Geometry check sheet. Reference: the model listing, model coordinates, mm. Face numbers are marked on the shaded views. A direction names the side the tool comes from. Coordinates: 2 decimals unless noted, no trailing zeros. Order: outer loops, then holes, each group sorted by start corner. A loop starts at its lowest first (then second) coordinate and runs counter-clockwise, first axis right, second up. Notation, with made-up numbers: (33.5, 70) - (86.5, 70) arc R29 cw to (86.5, 94) - close; hole circle Ø3 at (81, 68). An arc over 180 degrees is marked (long way). One line per item, written item: value. Start each with the question number.
```python
from build123d import *

# Parameters (mm, degrees)
SKETCH_W           = 18.5
SKETCH_H           = 18.5
SKETCH_R           = 8.15
PAD_DEPTH          = 4
SKETCH001_W        = 18.5
SKETCH001_H        = 18.5
PAD001_DEPTH       = 3
SKETCH002_R        = 9.25
SKETCH003_R        = 5.4
SKETCH005_R        = 5.4
PAD002_DEPTH       = 2
CHAMFER_SIZE       = 1.5
CHAMFER001_SIZE    = 1.5
POCKET_DEPTH       = 102.726887
POLARPATTERN_COUNT = 4
SKETCH007_R        = 4.4
SKETCH008_R        = 5.4
SKETCH009_W        = 9
SKETCH009_H        = 1
PAD003_DEPTH       = 1
SKETCH012_R        = 0.5655
SKETCH012_W        = 3.231
SKETCH012_H        = 0.497
POCKET001_DEPTH    = 18.501
POCKET002_DEPTH    = 13.751


with BuildPart() as part:
    # Sketch → Pad (new body)
    with BuildSketch(Plane.XY):
        Rectangle(SKETCH_W, SKETCH_H)
        Circle(SKETCH_R, mode=Mode.SUBTRACT)
    extrude(amount=PAD_DEPTH)

    # Sketch001 (on Face7 of Pad) → Pad001 (join)
    with BuildSketch(Plane.XY.offset(4)):
        Rectangle(SKETCH001_W, SKETCH001_H)
    extrude(amount=PAD001_DEPTH)

    # Sketch002 (on Face10 of Pad001) → AdditiveLoft section 0
    with BuildSketch(Plane.XY.offset(7)):
        Circle(SKETCH002_R)
    # Sketch003 (on Face10 of Pad001) → AdditiveLoft section 1
    with BuildSketch(Plane.XY.offset(31)):
        Circle(SKETCH003_R)
    loft()

    # Sketch005 (on Face17 of AdditiveLoft) → Pad002 (join)
    with BuildSketch(Plane.XY.offset(31)):
        Circle(SKETCH005_R)
    extrude(amount=PAD002_DEPTH)

    # Chamfer
    chamfer_edges = [part.edges().sort_by_distance(p)[0] for p in [
        (-9.25, -9.25, 5.5),
        (-9.25, -9.25, 2),
        (9.25, -9.25, 5.5),
        (9.25, -9.25, 2),
        (9.25, 9.25, 2),
        (9.25, 9.25, 5.5),
        (-9.25, 9.25, 5.5),
        (-9.25, 9.25, 2),
    ]]
    chamfer(chamfer_edges, length=CHAMFER_SIZE)

    # Chamfer001
    chamfer001_edges = [part.edges().sort_by_distance(p)[0] for p in [
        (8.5, -8.5, 7),
        (-8.5, -8.5, 7),
        (-8.5, 8.5, 7),
        (8.5, 8.5, 7),
    ]]
    chamfer(chamfer001_edges, length=CHAMFER001_SIZE)

    # Sketch006 (on Face19 of Chamfer001) → Pocket (cut, through all)
    with BuildSketch(Plane.YZ.offset(9.25)):
        Polygon((0, 31), (-2.7, 7), (2.7, 7), align=None)
    pocket = extrude(amount=-POCKET_DEPTH, mode=Mode.SUBTRACT)

    # PolarPattern: Pocket ×4 about axis
    polarpattern_axis = Axis((0, 0, 0), (0, 0, 1))
    for i in range(1, POLARPATTERN_COUNT):
        add(pocket.rotate(polarpattern_axis, i * 360 / POLARPATTERN_COUNT), mode=Mode.SUBTRACT)

    # Sketch007 (on Face47 of PolarPattern) → AdditiveLoft001 section 0
    with BuildSketch(Plane.XY.offset(33)):
        Circle(SKETCH007_R)
    # Sketch008 → AdditiveLoft001 section 1
    with BuildSketch(Plane.XY.offset(35)):
        Circle(SKETCH008_R)
    loft()

    # Sketch009 (on Face56 of AdditiveLoft001) → Pad003 (join)
    with BuildSketch(Plane.XY.offset(35)):
        Rectangle(SKETCH009_W, SKETCH009_H)
    extrude(amount=PAD003_DEPTH)

    # Sketch010 (on Face59 of Pad003) → AdditiveLoft002 section 0
    with BuildSketch(Plane.YZ.offset(4.5)):
        Polygon((-3, 35), (-4.75, 43), (4.75, 43), (3, 35), align=None)
    # Sketch011 → AdditiveLoft002 section 1
    with BuildSketch(Plane(origin=(-6, 0, 0), x_dir=(0, -1, 0), z_dir=(-1, 0, 0))):
        Polygon((-1.5, 37.4), (1.5, 37.4), (1, 35), (-1, 35), align=None)
    loft()

    # Sketch012 (on Face43 of AdditiveLoft002) → Pocket001 (cut, through all)
    with BuildSketch(Plane.XZ.offset(9.25)):
        with Locations((1.06, 38.921)):
            Circle(SKETCH012_R)
        with Locations((-4.9245, 36.0185)):
            Rectangle(SKETCH012_W, SKETCH012_H)
    extrude(amount=-POCKET001_DEPTH, mode=Mode.SUBTRACT)

    # Sketch013 (on Face62 of Pocket001) → Pocket002 (cut, through all)
    with BuildSketch(Plane.YZ.offset(4.5)):
        Polygon((0, 44.847), (5.530097, 43.207534), (0, 41.847), (-5.530097, 43.207534), align=None)
    extrude(amount=-POCKET002_DEPTH, mode=Mode.SUBTRACT)


solid = part.part
```
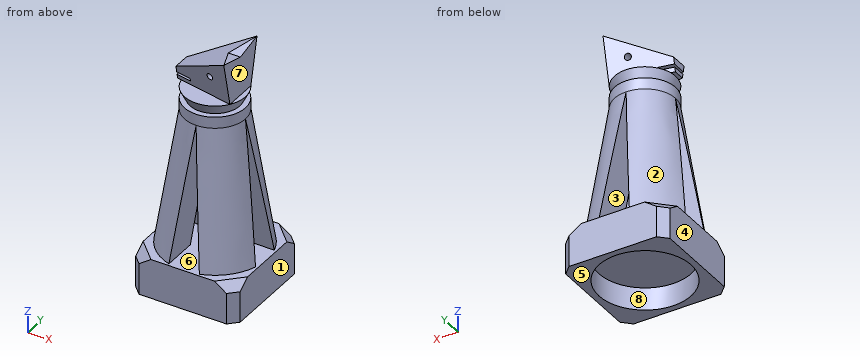
Q1. Material ranges on probe 1 along Y at (x, z) = (0, 3.2); probe 2 along Z at (x, y) = (5.5, 0); probe 3 along X at (y, z) = (5.25, 22.5), recorded low to high.
Q2. Cross-section at B-B, the plane y = 0.5. Count the separate pieces of the cut face and the enclosed holes in it, and give its area (3 significant figures).
Q3. Cross-section at C-C, the plane z = 33.5. Enter the section's corners in (x, y).
Q4. Gauge pin test, flat ends, axial feed: P1, Ø8, axis at x = 1.5, y = 3, coming from the -Z side; P2, Ø1.3, axis at x = -5, y = 0.5, coming from the +Z side; P3, Ø5.5, axis at x = 0, y = 0.5, coming from the +Z side; P4, Ø6, axis at x = 4.5, y = 2, coming from the +Z side. Record the tip position at first contact, or that the pin passes through.
Q5. Cross-section at A-A, the plane z = 18. Enter the section's corners in (x, y), and give its area (3 significant figures).
Q6. Set-up check for the marked faces 4, 5, 6, 7 and 8: record each of +Z, -Z, +X, -X, +Y, -Y from which the full face is reachable in a straight line by a thin tool's end or side.
Q7. Release check for a two-part mould opening along X. For the marked faces 1, 2 and 3 record: released by +X, released by -X, zero draft, split by the parting line, or undercut.
Check result:
1. probe 1: y = -9.25 to -8.15, 8.15 to 9.25
1. probe 2: z = 4 to 7
1. probe 3: x = -4.26 to -0.96, 0.96 to 4.26
2. separate pieces: 2
2. enclosed holes: 1
2. area: 205 mm2
3. outline: circle Ø9.3 at (0, 0)
4. P1: stops at z = 4
4. P2: stops at z = 38.28
4. P3: stops at z = 42.06
4. P4: stops at z = 43
5. outline: (-7.34, -1.46) arc R7.49 ccw to (-1.46, -7.34) - (-1.46, -1.46) - close; (-7.34, 1.46) - (-1.46, 1.46) - (-1.46, 7.34) arc R7.49 ccw to start; (1.46, -7.34) arc R7.49 ccw to (7.34, -1.46) - (1.46, -1.46) - close; (1.46, 1.46) - (7.34, 1.46) arc R7.49 ccw to (1.46, 7.34) - close
5. area: 97.6 mm2
6. face 4: +Z, -Z, -X, +Y, -Y
6. face 5: -Z, +X, -X, +Y, -Y
6. face 6: none
6. face 7: +Z, +X, +Y, -Y
6. face 8: -Z
7. face 1: released by +X
7. face 2: released by -X
7. face 3: undercut
